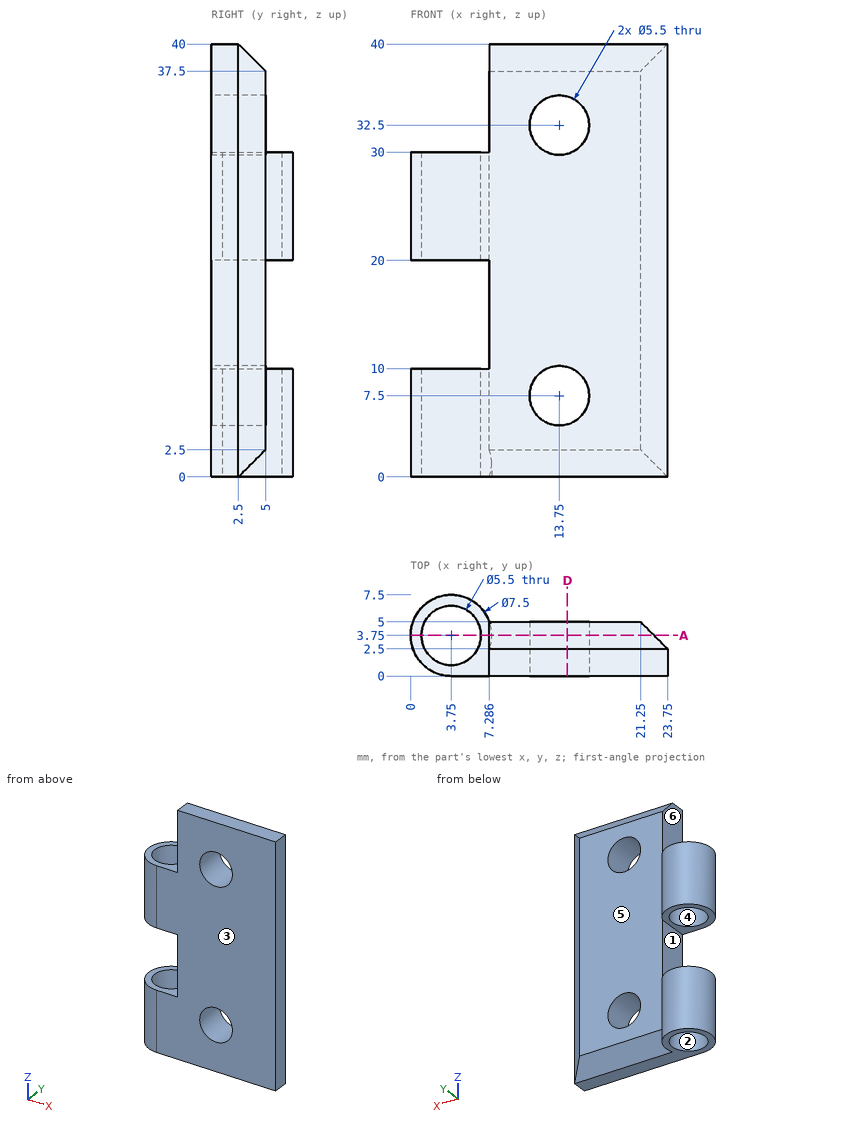
Can you work these out from the drawing? Everything is in mm from the part's minimum corner. A direction names the side the tool comes from. Coordinates: 2 decimals unless noted, no trailing zeros. Loops run counter-clockwise (first coordinate to the right, second up) from the corner with the lowest first, then second, coordinate; pieces in that order, holes last.
1) Thinking about a two-plate mould opening in Y: for the marked faces 1, 2 and 3, which applies, pulls with the +Y half, pulls with the -Y half, needs draft (parallel to the pull), parting line crosses it, or undercut?
2) I need wall thicknesses on probe 1 along Z at (x, y) = (13.75, 2.5); probe 2 along Z at (x, y) = (1.5, 1.75); probe 3 along X at (y, z) = (3.75, 27). Which ranges of each line are inside material? Lowest first, please.
3) For pin 1 (2 mm diameter, centred on y = 1, z = 20, fed in from -X); pin 2 (1.5 mm diameter, centred on y = 3.5, z = 36, fed in from -X); pin 3 (4 mm diameter, centred on x = 17, y = 5.5, fed in from +Z), each with a flat end and sliding along its axis, tell me the tip position at first contact or that it passes through.
4) Imagine slicing it at A-A on y = 3.75. State how many separate pieces and enclosed holes the cut face has, plus the area to 3 significant figures.
5) Imagine slicing it at D-D on x = 14.5. List the corners of the cut face in (y, z) for me (1 decimal).
6) Which directions (+Z, -Z, +X, -X, +Y, -Y) give clear straight access to the entire face, cutting with the end or side of a thin tool? Please do the marked faces 4, 5 and 6.
Completed:
1. face 1: needs draft
1. face 2: undercut
1. face 3: pulls with the -Y half
2. probe 1: z = 0 to 4.75, 10.25 to 29.75, 35.25 to 40
2. probe 2: z = 0 to 10, 20 to 30
2. probe 3: x = 0 to 1, 6.5 to 22.5
3. pin 1: stops at x = 0.43
3. pin 2: stops at x = 7.29
3. pin 3: stops at z = 39
4. separate pieces: 3
4. enclosed holes: 2
4. area: 559 mm2
5. outline: (0, 0) - (2.5, 0) - (5, 2.5) - (5, 4.9) - (0, 4.9) - close; (0, 10.1) - (5, 10.1) - (5, 29.9) - (0, 29.9) - close; (0, 35.1) - (5, 35.1) - (5, 37.5) - (2.5, 40) - (0, 40) - close
6. face 4: +Z, -Z
6. face 5: +Z, -Z, +X, +Y
6. face 6: +Z, -X, +Y, -Y
